Geometry: final body of the model. Coordinates: model frame, mm. A direction names the side the tool comes from. Round coordinates to 2 decimals unless told otherwise and drop trailing zeros. Order: outer loops, then holes, each group sorted by start corner. A loop starts at its lowest first (then second) coordinate and runs counter-clockwise, first axis right, second up. Notation, with made-up numbers: M 56.5,12.25 L 90.5,12.25 A18 cw 90.5,18.25 Z; hole C -24.5,-27 d4. An arc over 180 degrees is marked long. Return JSON: item names as keys, results as strings. Group by question number.
Q1. Mould query, pull axis Z, two halves, no side actions, for faces 1 (the face through (274.9, 5, 22)), 2 (the face through (172, 6, 102.515)), 3 (the face through (74, 3.175, 110)). Classes: released by +Z, released by -Z, zero draft, split by the parting line, or undercut.
Q2. Contact query for flat-ended pins moving along their axis: pin 1 (2.5 mm diameter, centred on y = 1, z = -62.5, fed in from -X); pin 2 (3.5 mm diameter, centred on y = 2, z = 107.5, fed in from +X); pin 3 (6.5 mm diameter, centred on x = 270.5, z = 109, fed in from +Y) (3 decimals); pin 4 (5 mm diameter, centred on x = 238, y = 11, fed in from -Z). Output: stop coordinate, or through.
Q3. Cut plane A-A on x = 189. Output: boundary loops of the cut face in (y, z) (3 decimals).
Q4. Cut plane C-C on z = -47.5. Output: boundary loops of the cut face in (x, y) (3 decimals).
Q5. Cut plane B-B on z = 62. Output: boundary loops of the cut face in (x, y) (3 decimals), and give its area (3 significant figures).
Q6. Access query for faces 4 (the face through (68.271, 6, 22)), 5 (the face through (172, 12.7, 93)), 6 (the face through (74, 3.175, -64)), 7 (the face through (272, 3.175, 110)), 8 (the face through (172, 9.525, 90)). Directions: +Z, -Z, +X, -X, +Y, -Y. A direction counts if a zero-diameter tool reaches every point of the face in a straight line with its end or side. Return the directions, or none.
Q7. Ray query, probe 1 along X at (y, z) = (9.75, 21); probe 2 along X at (y, z) = (1, 88); probe 3 along Z at (x, y) = (116, 9). Return the intervals inside material, ascending.
```python
from build123d import *

# Parameters (mm, degrees)
SKETCH1_W               = 209.55
SKETCH1_H               = 158.75
SKETCH1_W_2             = 177.8
SKETCH1_H_2             = 127
FRONTFACE_DEPTH         = 3.175
SKETCH3_W               = 209.55
SKETCH3_H               = 158.75
SKETCH3_W_2             = 203.708
SKETCH3_H_2             = 152.908
SIDESHELL_DEPTH         = 9.525
BOTTOMSUPPORTLOCK_DEPTH = 3.175
FILLET1_R               = 2.54


with BuildPart() as part:
    # Sketch1 → FrontFace (new body)
    with BuildSketch(Plane(origin=(0, 9.525, 0), x_dir=(1, 0, 0), z_dir=(0, 1, 0))):
        with Locations((173.045515995, -23.140372536)):
            Rectangle(SKETCH1_W, SKETCH1_H)
        with Locations((173.045515995, -23.140372536)):
            Rectangle(SKETCH1_W_2, SKETCH1_H_2, mode=Mode.SUBTRACT)
    extrude(amount=FRONTFACE_DEPTH)

    # Sketch3 → SideShell (add)
    with BuildSketch(Plane.XZ.offset(-9.525)):
        with Locations((173.045515995, 23.140372536)):
            Rectangle(SKETCH3_W, SKETCH3_H)
        with Locations((173.045515995, 23.140372536)):
            Rectangle(SKETCH3_W_2, SKETCH3_H_2, mode=Mode.SUBTRACT)
    extrude(amount=SIDESHELL_DEPTH)

    # Sketch9 → BottomSupportLock (add)
    with BuildSketch(Plane.XZ):
        with BuildLine():
            Line((277.820515995, 102.515372536), (268.036564976, 102.515372536))
            Line((268.036564976, 102.515372536), (268.036564976, 113.237616687))
            Line((268.036564976, 113.237616687), (277.820515995, 113.237616687))
            Line((277.820515995, 113.237616687), (277.820515995, 109.721147351))
            ThreePointArc((277.820515995, 109.721147351), (277.744362054, 109.539800226), (277.561564976, 109.467195608))
            Line((277.561564976, 109.467195608), (271.211564976, 109.590994612))
            Line((271.211564976, 109.590994612), (271.211564976, 106.161994612))
            Line((271.211564976, 106.161994612), (277.520350721, 106.282567338))
            ThreePointArc((277.520350721, 106.282567338), (277.702016533, 106.210968908), (277.779186707, 106.031598992))
            Line((277.779186707, 106.031598992), (277.820515995, 102.515372536))
        make_face()
        with BuildLine():
            Line((277.779186707, -59.750853919), (277.820515995, -56.234627464))
            Line((277.820515995, -56.234627464), (268.036564976, -56.234627464))
            Line((268.036564976, -56.234627464), (268.036564976, -66.956871614))
            Line((268.036564976, -66.956871614), (277.820515995, -66.956871614))
            Line((277.820515995, -66.956871614), (277.820515995, -63.440402278))
            ThreePointArc((277.820515995, -63.440402278), (277.744362054, -63.259055154), (277.561564976, -63.186450536))
            Line((277.561564976, -63.186450536), (271.211564976, -63.310249539))
            Line((271.211564976, -63.310249539), (271.211564976, -59.881249539))
            Line((271.211564976, -59.881249539), (277.520350721, -60.001822265))
            ThreePointArc((277.520350721, -60.001822265), (277.702016533, -59.930223835), (277.779186707, -59.750853919))
        make_face()
        with BuildLine():
            Line((68.270515995, -56.234627464), (78.054467015, -56.234627464))
            Line((78.054467015, -56.234627464), (78.054467015, -66.956871614))
            Line((78.054467015, -66.956871614), (68.270515995, -66.956871614))
            Line((68.270515995, -66.956871614), (68.270515995, -63.440402278))
            ThreePointArc((68.270515995, -63.440402278), (68.346669937, -63.259055154), (68.529467015, -63.186450536))
            Line((68.529467015, -63.186450536), (74.879467015, -63.310249539))
            Line((74.879467015, -63.310249539), (74.879467015, -59.881249539))
            Line((74.879467015, -59.881249539), (68.57068127, -60.001822265))
            ThreePointArc((68.57068127, -60.001822265), (68.389015458, -59.930223835), (68.311845284, -59.750853919))
            Line((68.311845284, -59.750853919), (68.270515995, -56.234627464))
        make_face()
        with BuildLine():
            Line((68.311845284, 106.031598992), (68.270515995, 102.515372536))
            Line((68.270515995, 102.515372536), (78.054467015, 102.515372536))
            Line((78.054467015, 102.515372536), (78.054467015, 113.237616687))
            Line((78.054467015, 113.237616687), (68.270515995, 113.237616687))
            Line((68.270515995, 113.237616687), (68.270515995, 109.721147351))
            ThreePointArc((68.270515995, 109.721147351), (68.346669937, 109.539800226), (68.529467015, 109.467195608))
            Line((68.529467015, 109.467195608), (74.879467015, 109.590994612))
            Line((74.879467015, 109.590994612), (74.879467015, 106.161994612))
            Line((74.879467015, 106.161994612), (68.57068127, 106.282567338))
            ThreePointArc((68.57068127, 106.282567338), (68.389015458, 106.210968908), (68.311845284, 106.031598992))
        make_face()
    extrude(amount=-BOTTOMSUPPORTLOCK_DEPTH)

    # Fillet1
    fillet1_edges = [part.edges().sort_by_distance(p)[0] for p in [
        (73.162491505, 3.175, 102.515372536),
        (78.054467015, 1.5875, 102.515372536),
        (272.928540486, 3.175, 102.515372536),
        (268.036564976, 1.5875, 102.515372536),
        (272.928540486, 3.175, -56.234627464),
        (268.036564976, 1.5875, -56.234627464),
        (73.162491505, 3.175, -56.234627464),
        (78.054467015, 1.5875, -56.234627464),
    ]]
    fillet(fillet1_edges, radius=FILLET1_R)


solid = part.part
```
Result sheet:
{
 "1": {"face 1": "undercut", "face 2": "released by +Z", "face 3": "zero draft"},
 "2": {"pin 1": "stops at x = 68.27", "pin 2": "stops at x = 277.78", "pin 3": "stops at y = 3.175", "pin 4": "stops at z = -56.23"},
 "3": {"outline": "M 0,-56.235 L 12.7,-56.235 L 12.7,-40.36 L 9.525,-40.36 L 9.525,-53.314 L 0,-53.314 Z; M 0,99.594 L 9.525,99.594 L 9.525,86.64 L 12.7,86.64 L 12.7,102.515 L 0,102.515 Z"},
 "4": {"outline": "M 68.271,0 L 71.192,0 L 71.192,9.525 L 274.9,9.525 L 274.9,0 L 277.821,0 L 277.821,12.7 L 68.271,12.7 Z"},
 "5": {"outline": "M 68.271,0 L 71.192,0 L 71.192,9.525 L 84.146,9.525 L 84.146,12.7 L 68.271,12.7 Z; M 261.946,9.525 L 274.9,9.525 L 274.9,0 L 277.821,0 L 277.821,12.7 L 261.946,12.7 Z", "area": "156 mm²"},
 "6": {"face 4": "+Z, -Z, -X, +Y, -Y", "face 5": "+Z, -Z, +X, -X, +Y", "face 6": "-Z, +X, -X, +Y", "face 7": "+Z, +X, -X, +Y", "face 8": "-Y"},
 "7": {"probe 1": "x = 68.27 to 84.15, 261.95 to 277.82", "probe 2": "x = 68.27 to 71.19, 274.9 to 277.82", "probe 3": "z = -56.23 to -53.31, 99.59 to 102.52"}
}
